Check sheet for the modelled part. Datum: model origin and axes. Units: mm. Coordinates: 2 decimals unless noted, no trailing zeros. Write each loop counter-clockwise with the first axis right and the second up, starting at its lowest first coordinate (ties: lowest second). Pieces come first, ordered by that corner, then holes. Notation, with made-up numbers: (-5, 42.25) - (36, 42.25) arc R6 cw to (36, 52.25) - close; hole circle Ø2 at (11.5, 45.5). An arc over 180 degrees is marked (long way). Write each question's results on one line, items separated by ' | '.
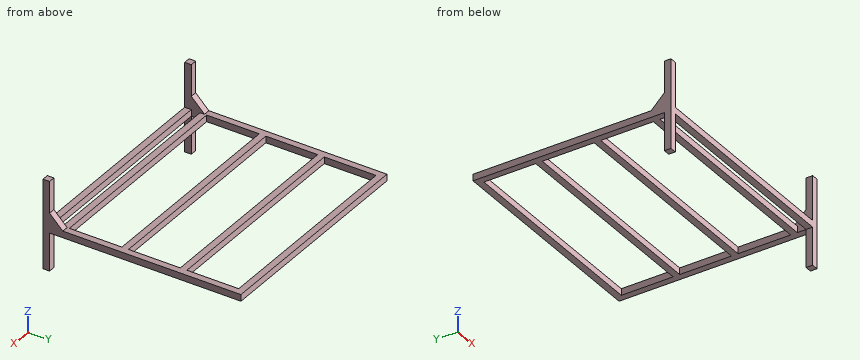
from build123d import *

# Parameters (mm, degrees)
SKETCH1_W           = 1010
SKETCH1_H           = 900
SKETCH1_W_2         = 950
SKETCH1_H_2         = 840
SKETCH1_H_3         = 30
BOSS_EXTRUDE1_DEPTH = 30
SKETCH2_W           = 30
SKETCH2_H           = 30
BOSS_EXTRUDE2_DEPTH = 203
SKETCH3_W           = 30
SKETCH3_H           = 30
BOSS_EXTRUDE3_DEPTH = 172
BOSS_EXTRUDE4_DEPTH = 30
BOSS_EXTRUDE5_DEPTH = 30


with BuildPart() as part:
    # Sketch1 → Boss-Extrude1 (new body)
    # profile 1 of 4: a face of its own
    with BuildSketch(Plane.XY):
        with Locations((505, -450)):
            Rectangle(SKETCH1_W, SKETCH1_H)
        with Locations((505, -450)):
            Rectangle(SKETCH1_W_2, SKETCH1_H_2, mode=Mode.SUBTRACT)
    # profile 2 of 4: a face of its own
    with BuildSketch(Plane.XY):
        with Locations((505, -815)):
            Rectangle(SKETCH1_W_2, SKETCH1_H_3)
    # profile 3 of 4: a face of its own
    with BuildSketch(Plane.XY):
        with Locations((505, -546)):
            Rectangle(SKETCH1_W_2, SKETCH1_H_3)
    # profile 4 of 4: a face of its own
    with BuildSketch(Plane.XY):
        with Locations((505, -280.5)):
            Rectangle(SKETCH1_W_2, SKETCH1_H_3)
    extrude(amount=BOSS_EXTRUDE1_DEPTH)

    # Sketch2 → Boss-Extrude2 (add)
    with BuildSketch(Plane.XY.offset(30)):
        with Locations((15, -885)):
            Rectangle(SKETCH2_W, SKETCH2_H)
        with Locations((995, -885)):
            Rectangle(SKETCH2_W, SKETCH2_H)
    extrude(amount=BOSS_EXTRUDE2_DEPTH)

    # Sketch3 → Boss-Extrude3 (add)
    with BuildSketch(Plane(origin=(0, 0, 0), x_dir=(-1, 0, 0), z_dir=(0, 0, -1))):
        with Locations((-15, -885)):
            Rectangle(SKETCH3_W, SKETCH3_H)
        with Locations((-995, -885)):
            Rectangle(SKETCH3_W, SKETCH3_H)
    extrude(amount=BOSS_EXTRUDE3_DEPTH)

    # Sketch4 → Boss-Extrude4 (add)
    with BuildSketch(Plane.ZY):
        Polygon((30, -810), (90, -870), (30, -870), align=None)
    extrude(amount=-BOSS_EXTRUDE4_DEPTH)

    # Sketch5 → Boss-Extrude5 (add)
    with BuildSketch(Plane(origin=(1010, 0, 0), x_dir=(0, 0, -1), z_dir=(1, 0, 0))):
        Polygon((-30, -810), (-30, -870), (-90, -870), align=None)
    extrude(amount=-BOSS_EXTRUDE5_DEPTH)


solid = part.part
1. Go/stop test with a flat-tipped pin: pin 1 (24 mm diameter, centred on x = 997.5, z = 157, fed in from +Y). Record where the tip stops, or that it passes through.
Values follow:
pin 1: stops at y = -870
2. Sectioned sample at B-B (x = 454). Record the cut outline in (y, z).
Values follow:
outline: (-900, 0) - (-870, 0) - (-870, 30) - (-900, 30) - close; (-830, 0) - (-800, 0) - (-800, 30) - (-830, 30) - close; (-561, 0) - (-531, 0) - (-531, 30) - (-561, 30) - close; (-295.5, 0) - (-265.5, 0) - (-265.5, 30) - (-295.5, 30) - close; (-30, 0) - (0, 0) - (0, 30) - (-30, 30) - close
3. Material ranges on L1, parallel to Y at x = 239, z = 15, recorded low to high. Write a range as [from, to].
Values follow:
L1: y = [-900, -870], [-830, -800], [-561, -531], [-295.5, -265.5], [-30, 0]
4. Sectioned sample at A-A (z = 54). Record the cut outline in (x, y).
Values follow:
outline: (0, -900) - (30, -900) - (30, -834) - (0, -834) - close; (980, -900) - (1010, -900) - (1010, -834) - (980, -834) - close
5. Sectioned sample at C-C (y = -482). Record the cut outline in (x, z), then the cut area to 3 significant figures.
Values follow:
outline: (0, 0) - (30, 0) - (30, 30) - (0, 30) - close; (980, 0) - (1010, 0) - (1010, 30) - (980, 30) - close | area: 1,800 mm^2
